```python
from build123d import *

# Parameters (mm, degrees)
CROQUIS1_W              = 135
CROQUIS1_H              = 30
SALIENTE_EXTRUIR1_DEPTH = 10
REDONDEO3_R             = 10
CROQUIS3_R              = 1.5
CROQUIS3_R_2            = 3.5
CORTAR_EXTRUIR2_DEPTH   = 10
SALIENTE_EXTRUIR2_START = 5
CROQUIS4_R              = 6
CROQUIS4_R_2            = 3.5
SALIENTE_EXTRUIR2_DEPTH = 5
CROQUIS5_R              = 1
CORTAR_EXTRUIR3_DEPTH   = 6


with BuildPart() as part:
    # Croquis1 → Saliente-Extruir1 (new body)
    with BuildSketch(Plane(origin=(0, 0, 0), x_dir=(1, 0, 0), z_dir=(0, 1, 0))):
        Rectangle(CROQUIS1_W, CROQUIS1_H)
    extrude(amount=SALIENTE_EXTRUIR1_DEPTH)

    # Redondeo3
    redondeo3_edges = [part.edges().sort_by_distance(p)[0] for p in [
        (-67.5, 5, -15),
        (67.5, 5, -15),
        (67.5, 5, 15),
        (-67.5, 5, 15),
    ]]
    fillet(redondeo3_edges, radius=REDONDEO3_R)

    # Croquis3 → Cortar-Extruir2 (cut)
    with BuildSketch(Plane(origin=(0, 10, 0), x_dir=(1, 0, 0), z_dir=(0, 1, 0))):
        with Locations(Location((-57.5, 0, 0), (0, 0, 270))):
            Circle(CROQUIS3_R)
        with Locations(Location((56.5, 0, 0), (0, 0, 270))):
            Circle(CROQUIS3_R_2)
    extrude(amount=-CORTAR_EXTRUIR2_DEPTH, mode=Mode.SUBTRACT)

    # Croquis4 → Saliente-Extruir2 (add)
    with BuildSketch(Plane(origin=(0, 10, 0), x_dir=(1, 0, 0), z_dir=(0, 1, 0)).offset(SALIENTE_EXTRUIR2_START)):
        with Locations(Location((56.5, 0, 0), (0, 0, 270))):
            Circle(CROQUIS4_R)
        with Locations(Location((56.5, 0, 0), (0, 0, 270))):
            Circle(CROQUIS4_R_2, mode=Mode.SUBTRACT)
    extrude(amount=-SALIENTE_EXTRUIR2_DEPTH)

    # Croquis5 → Cortar-Extruir3 (cut)
    with BuildSketch(Plane(origin=(56.5, 0, 0), x_dir=(0, 0, -1), z_dir=(1, 0, 0))):
        with Locations(Location((0, 12.5, 0), (0, 0, 180))):
            Circle(CROQUIS5_R)
    extrude(amount=CORTAR_EXTRUIR3_DEPTH, mode=Mode.SUBTRACT)


solid = part.part
```
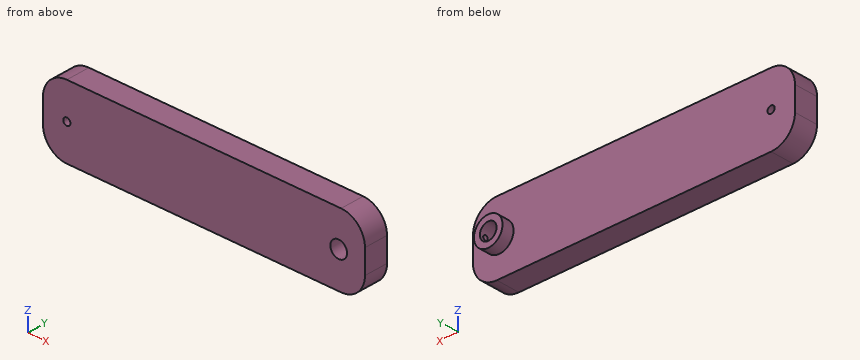
Design review of the part built by this model. Coordinates are the model's own, in mm. Coordinates: 2 decimals unless noted, no trailing zeros. Write each loop counter-clockwise with the first axis right and the second up, starting at its lowest first coordinate (ties: lowest second). Pieces come first, ordered by that corner, then holes. Notation, with made-up numbers: M -14.75,51.5 L 39.25,51.5 A20 ccw 39.25,82.5 Z; hole C 81,55 d4. An arc over 180 degrees is marked long. Answer as a JSON object with one key per item and string values.
Item 1: Add section C-C, the plane z = 8.5. Give the boundary of the cut face in (x, y).
Outcome:
{"outline": "M -66.87,0 L 66.87,0 L 66.87,10 L -66.87,10 Z"}
Item 2: Add section A-A, the plane y = 8. Give the boundary of the cut face in (x, z).
Outcome:
{"outline": "M -67.5,-5 A10 ccw -57.5,-15 L 57.5,-15 A10 ccw 67.5,-5 L 67.5,5 A10 ccw 57.5,15 L -57.5,15 A10 ccw -67.5,5 Z; hole C -57.5,0 d3; hole C 56.5,0 d7"}
Item 3: Wall thickness on probe 1 along X at (y, z) = (6, 0); probe 2 along Y at (x, z) = (61.4, 0); probe 3 along Y at (x, z) = (7.5, -8.5): over which ranges is each line inside the solid? List them lowest first.
Outcome:
{"probe 1": "-67.5 to -59, -56 to 53, 60 to 67.5", "probe 2": "0 to 11.5, 13.5 to 15", "probe 3": "0 to 10"}
Item 4: Add section B-B, the plane x = -21.5. Give the boundary of the cut face in (y, z).
Outcome:
{"outline": "M 0,-15 L 10,-15 L 10,15 L 0,15 Z"}
Item 5: Insertion check: pin 1 Ø1.6 at (y, z) = (12.5, 0) entering from +X; pin 2 Ø3 at (y, z) = (7.5, -10) entering from +X; pin 3 Ø1.8 at (x, z) = (-57.5, 0) entering from +Y; pin 4 Ø9 at (x, z) = (-12.5, -5) entering from +Y. Each pin has a flat end and moves straight along its axis. Give the tip position at first contact, or say it passes through.
Outcome:
{"pin 1": "x = 53.09", "pin 2": "x = 66.87", "pin 3": "through", "pin 4": "y = 10"}
